```python
from build123d import *

# Parameters (mm, degrees)
SKETCH2_W           = 43.72
SKETCH2_H           = 43.72
SKETCH2_W_2         = 37.72
SKETCH2_H_2         = 37.72
BOSS_EXTRUDE1_DEPTH = 5
SKETCH1_R           = 0.95
CUT_EXTRUDE1_DEPTH  = 6


with BuildPart() as part:
    # Sketch2 → Boss-Extrude1 (new body)
    with BuildSketch(Plane(origin=(0, 0, 0), x_dir=(1, 0, 0), z_dir=(0, 1, 0))):
        Rectangle(SKETCH2_W, SKETCH2_H)
        Rectangle(SKETCH2_W_2, SKETCH2_H_2, mode=Mode.SUBTRACT)
    extrude(amount=BOSS_EXTRUDE1_DEPTH)

    # Sketch1 → Cut-Extrude1 (cut, through all)
    with BuildSketch(Plane(origin=(0, 0, 0), x_dir=(1, 0, 0), z_dir=(0, 1, 0))):
        with Locations((-20.269, -20.269)):
            Circle(SKETCH1_R)
        with Locations((-17.879, -20.269)):
            Circle(SKETCH1_R)
        with Locations((-15.489, -20.269)):
            Circle(SKETCH1_R)
        with Locations((-13.099, -20.269)):
            Circle(SKETCH1_R)
        with Locations((-10.709, -20.269)):
            Circle(SKETCH1_R)
        with Locations((-8.319, -20.269)):
            Circle(SKETCH1_R)
        with Locations((-5.929, -20.269)):
            Circle(SKETCH1_R)
        with Locations((-3.539, -20.269)):
            Circle(SKETCH1_R)
        with Locations((-1.149, -20.269)):
            Circle(SKETCH1_R)
        with Locations((1.241, -20.269)):
            Circle(SKETCH1_R)
        with Locations((3.631, -20.269)):
            Circle(SKETCH1_R)
        with Locations((6.021, -20.269)):
            Circle(SKETCH1_R)
        with Locations((8.411, -20.269)):
            Circle(SKETCH1_R)
        with Locations((10.801, -20.269)):
            Circle(SKETCH1_R)
        with Locations((13.191, -20.269)):
            Circle(SKETCH1_R)
        with Locations((20.269, 20.269)):
            Circle(SKETCH1_R)
        with Locations((20.269, -15.581)):
            Circle(SKETCH1_R)
        with Locations((20.269, -13.191)):
            Circle(SKETCH1_R)
        with Locations((20.269, -10.801)):
            Circle(SKETCH1_R)
        with Locations((20.269, -8.411)):
            Circle(SKETCH1_R)
        with Locations((20.269, -6.021)):
            Circle(SKETCH1_R)
        with Locations((20.269, -3.631)):
            Circle(SKETCH1_R)
        with Locations((20.269, -1.241)):
            Circle(SKETCH1_R)
        with Locations((20.269, 1.149)):
            Circle(SKETCH1_R)
        with Locations((20.269, 3.539)):
            Circle(SKETCH1_R)
        with Locations((20.269, 5.929)):
            Circle(SKETCH1_R)
        with Locations((20.269, 8.319)):
            Circle(SKETCH1_R)
        with Locations((20.269, 10.709)):
            Circle(SKETCH1_R)
        with Locations((20.269, 13.099)):
            Circle(SKETCH1_R)
        with Locations((20.269, 15.489)):
            Circle(SKETCH1_R)
        with Locations((20.269, 17.879)):
            Circle(SKETCH1_R)
        with Locations((13.159, 20.269)):
            Circle(SKETCH1_R)
        with Locations((10.769, 20.269)):
            Circle(SKETCH1_R)
        with Locations((8.379, 20.269)):
            Circle(SKETCH1_R)
        with Locations((5.989, 20.269)):
            Circle(SKETCH1_R)
        with Locations((3.599, 20.269)):
            Circle(SKETCH1_R)
        with Locations((1.209, 20.269)):
            Circle(SKETCH1_R)
        with Locations((-1.181, 20.269)):
            Circle(SKETCH1_R)
        with Locations((-3.571, 20.269)):
            Circle(SKETCH1_R)
        with Locations((-5.961, 20.269)):
            Circle(SKETCH1_R)
        with Locations((-8.351, 20.269)):
            Circle(SKETCH1_R)
        with Locations((-10.741, 20.269)):
            Circle(SKETCH1_R)
        with Locations((-13.131, 20.269)):
            Circle(SKETCH1_R)
        with Locations((-15.521, 20.269)):
            Circle(SKETCH1_R)
        with Locations((-17.911, 20.269)):
            Circle(SKETCH1_R)
        with Locations((-20.269, 20.301)):
            Circle(SKETCH1_R)
        with Locations((-20.269, 17.911)):
            Circle(SKETCH1_R)
        with Locations((-20.269, 15.521)):
            Circle(SKETCH1_R)
        with Locations((-20.269, 13.131)):
            Circle(SKETCH1_R)
        with Locations((-20.269, 10.741)):
            Circle(SKETCH1_R)
        with Locations((-20.269, 8.351)):
            Circle(SKETCH1_R)
        with Locations((-20.269, 5.961)):
            Circle(SKETCH1_R)
        with Locations((-20.269, 3.571)):
            Circle(SKETCH1_R)
        with Locations((-20.269, 1.181)):
            Circle(SKETCH1_R)
        with Locations((-20.269, -1.209)):
            Circle(SKETCH1_R)
        with Locations((-20.269, -3.599)):
            Circle(SKETCH1_R)
        with Locations((-20.269, -5.989)):
            Circle(SKETCH1_R)
        with Locations((-20.269, -8.379)):
            Circle(SKETCH1_R)
        with Locations((-20.269, -10.769)):
            Circle(SKETCH1_R)
        with Locations((-20.269, -13.159)):
            Circle(SKETCH1_R)
        with Locations((-20.269, -15.519)):
            Circle(SKETCH1_R)
        with Locations((-20.269, -17.879)):
            Circle(SKETCH1_R)
        with Locations((15.519, 20.269)):
            Circle(SKETCH1_R)
        with Locations((17.879, 20.269)):
            Circle(SKETCH1_R)
        with Locations((20.269, -17.941)):
            Circle(SKETCH1_R)
        with Locations((20.269, -20.301)):
            Circle(SKETCH1_R)
        with Locations((17.909, -20.301)):
            Circle(SKETCH1_R)
        with Locations((15.549, -20.301)):
            Circle(SKETCH1_R)
    extrude(amount=CUT_EXTRUDE1_DEPTH, mode=Mode.SUBTRACT)


solid = part.part
```
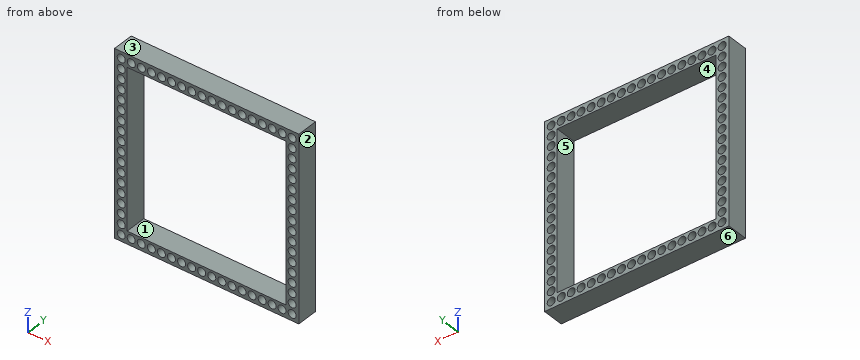
Can you work these out from the model? Positions are in its coordinate system, mm. Face numbers are marked on the shaded views. A direction names the side the tool comes from. Coordinates: 2 decimals unless noted, no trailing zeros. Loops run counter-clockwise (first coordinate to the right, second up) from the corner with the lowest first, then second, coordinate; pieces in that order, holes last. Notation, with made-up numbers: (39, 60.5) -> (66, 60.5) arc R30 ccw to (66, 90.5) -> close; hole circle Ø9 at (35.5, -16.75). An arc over 180 degrees is marked (long way). Answer as a JSON object with one key per item and string values.
1) Imagine slicing it at B-B (x = 1.5). Please give me the cut outline in (y, z), then the cut area to 3 significant figures.
Results:
{"outline": "(0, -21.86) -> (5, -21.86) -> (5, -21.17) -> (0, -21.17) -> close; (0, -19.36) -> (5, -19.36) -> (5, -18.86) -> (0, -18.86) -> close; (0, 18.86) -> (5, 18.86) -> (5, 19.35) -> (0, 19.35) -> close; (0, 21.18) -> (5, 21.18) -> (5, 21.86) -> (0, 21.86) -> close", "area": "11.8 mm^2"}
2) For P1, Ø1.1, axis at x = -20.269, z = -8.351, coming from the +Y side, with a flat end and sliding along its axis, tell me the tip position at first contact or that it passes through.
Results:
{"P1": "passes through"}
3) Imagine slicing it at C-C (y = 3.35). Count the separate pieces of the cut face and the enclosed holes in it, then the cut area to 3 significant figures.
Results:
{"separate pieces": "1", "enclosed holes": "69", "area": "296 mm^2"}
4) If I drill on line 1 (X direction, y = 3.15, z = 15.5); line 2 (X direction, y = 3.25, z = 5); line 3 (Z direction, x = -16, y = 0.4), over which ranges is the centre line in solid material (lowest first)?
Results:
{"line 1": "x = -21.86 to -21.22, -19.32 to -18.86, 18.86 to 19.32, 21.22 to 21.86", "line 2": "x = -21.86 to -18.86, 18.86 to 21.86", "line 3": "z = -21.86 to -21.09, -19.45 to -18.86, 18.86 to 19.47, 21.07 to 21.86"}
5) For the marked faces 5 and 6, which set-ups out of +Z, -Z, +X, -X, +Y, -Y let a thin tool reach every point of the face, with its end or its side?
Results:
{"face 5": "+Y, -Y", "face 6": "-Z, +X, -X, +Y, -Y"}
6) Thinking about a two-plate mould opening in Z: for the marked faces 1, 2, 3 and 4, which applies, pulls with the +Z half, pulls with the -Z half, needs draft (parallel to the pull), parting line crosses it, or undercut?
Results:
{"face 1": "undercut", "face 2": "needs draft", "face 3": "pulls with the +Z half", "face 4": "undercut"}
7) Imagine slicing it at A-A (x = -10.5). Please give me the cut outline in (y, z), then the cut area to 3 significant figures.
Results:
{"outline": "(0, -21.86) -> (5, -21.86) -> (5, -21.19) -> (0, -21.19) -> close; (0, -19.35) -> (5, -19.35) -> (5, -18.86) -> (0, -18.86) -> close; (0, 18.86) -> (5, 18.86) -> (5, 19.34) -> (0, 19.34) -> close; (0, 21.2) -> (5, 21.2) -> (5, 21.86) -> (0, 21.86) -> close", "area": "11.5 mm^2"}
